Input: part model. Units: mm. Frame: model coordinates. Face numbers are marked on the shaded views. Coordinates: 2 decimals unless noted, no trailing zeros. Loops run counter-clockwise (first coordinate to the right, second up) from the corner with the lowest first, then second, coordinate; pieces in that order, holes last. Notation, with made-up numbers: (46.5, 26) -> (88.5, 26) arc R16 ccw to (88.5, 32) -> close; hole circle Ø3 at (29, 40). An arc over 180 degrees is marked (long way). Answer as a JSON object with one key per item and string values.
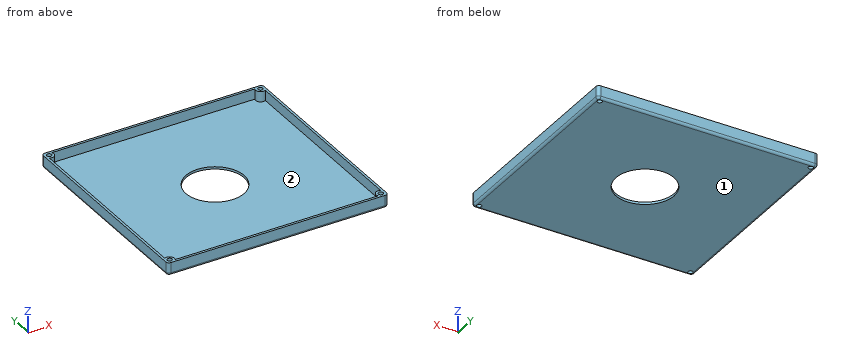
from build123d import *

# Parameters (mm, degrees)
SKETCH1_W                = 140
SKETCH1_H                = 133
BOSS_EXTRUDE1_DEPTH      = 8
F_3_0_3_DIAMETER_HOLE1_D = 3
SHELL3_T                 = -1.5
FILLET2_R                = 2
FILLET3_R                = 2
FILLET4_R                = 2
FILLET5_R                = 2
SKETCH13_R               = 18.454910332
CUT_EXTRUDE1_DEPTH       = 10
FILLET6_R                = 1.5


with BuildPart() as part:
    # Sketch1 → Boss-Extrude1 (new body)
    with BuildSketch(Plane.XY):
        Rectangle(SKETCH1_W, SKETCH1_H)
    extrude(amount=BOSS_EXTRUDE1_DEPTH)

    # Ø3.0 (3) Diameter Hole1 (through all)
    with Locations(Plane.XY.offset(8)):
        with Locations((-67, 63.5), (67, 63.5), (-67, -63.5), (67, -63.5)):
            Hole(F_3_0_3_DIAMETER_HOLE1_D / 2)

    # Shell3
    shell3_openings = [part.faces().sort_by_distance(p)[0] for p in [
        (0, 0, 8),
    ]]
    offset(amount=SHELL3_T, openings=shell3_openings)

    # Fillet2
    fillet2_edges = [part.edges().sort_by_distance(p)[0] for p in [
        (-70, 66.5, 4),
    ]]
    fillet(fillet2_edges, radius=FILLET2_R)

    # Fillet3
    fillet3_edges = [part.edges().sort_by_distance(p)[0] for p in [
        (-70, -66.5, 4),
    ]]
    fillet(fillet3_edges, radius=FILLET3_R)

    # Fillet4
    fillet4_edges = [part.edges().sort_by_distance(p)[0] for p in [
        (70, -66.5, 4),
    ]]
    fillet(fillet4_edges, radius=FILLET4_R)

    # Fillet5
    fillet5_edges = [part.edges().sort_by_distance(p)[0] for p in [
        (70, 66.5, 4),
    ]]
    fillet(fillet5_edges, radius=FILLET5_R)

    # Sketch13 → Cut-Extrude1 (cut)
    with BuildSketch(Plane(origin=(0, 0, 0), x_dir=(-1, 0, 0), z_dir=(0, 0, -1))):
        Circle(SKETCH13_R)
    extrude(amount=-CUT_EXTRUDE1_DEPTH, mode=Mode.SUBTRACT)

    # Fillet6
    fillet6_edges = [part.edges().sort_by_distance(p)[0] for p in [
        (-70, 0, 0),
        (-69.414213562, 65.914213562, 0),
        (0, -66.5, 0),
        (-69.414213562, -65.914213562, 0),
        (70, 0, 0),
        (69.414213562, -65.914213562, 0),
        (0, 66.5, 0),
        (69.414213562, 65.914213562, 0),
    ]]
    fillet(fillet6_edges, radius=FILLET6_R - 0.0001)  # a hair under: the kernel refuses the full size


solid = part.part
1. Section query A-A (y = -30). Return loops of the section in (x, z), plus the area to 3 significant figures.
Reply:
{"outline": "(-70, 1.5) arc R1.5 ccw to (-68.5, 0) -> (68.5, 0) arc R1.5 ccw to (70, 1.5) -> (70, 8) -> (68.5, 8) -> (68.5, 1.5) -> (-68.5, 1.5) -> (-68.5, 8) -> (-70, 8) -> close", "area": "229 mm2"}
2. Pin query (flat end, axial travel): P1, Ø22, axis at x = 0, y = 0, coming from the +Z side. Return the tip coordinate at first contact, or that it passes through.
Reply:
{"P1": "passes through"}
3. Section query D-D (x = 42.5). Return loops of the section in (y, z), plus the area to 3 significant figures.
Reply:
{"outline": "(-66.5, 1.5) arc R1.5 ccw to (-65, 0) -> (65, 0) arc R1.5 ccw to (66.5, 1.5) -> (66.5, 8) -> (65, 8) -> (65, 1.5) -> (-65, 1.5) -> (-65, 8) -> (-66.5, 8) -> close", "area": "218 mm2"}
4. Line query: line 1 along Y through (x, z) = (67, 2.75); line 2 along X through (y, z) = (-10.5, 4); line 3 along Y through (x, z) = (-19.5, 4.25). Output: solid intervals per line, ascending.
Reply:
{"line 1": "y = -66.5 to -65, -62 to -60.5, 60.5 to 62, 65 to 66.5", "line 2": "x = -70 to -68.5, 68.5 to 70", "line 3": "y = -66.5 to -65, 65 to 66.5"}
5. Section query B-B (z = 6.5). Return loops of the section in (x, y).
Reply:
{"outline": "(-70, -64.5) arc R2 ccw to (-68, -66.5) -> (68, -66.5) arc R2 ccw to (70, -64.5) -> (70, 64.5) arc R2 ccw to (68, 66.5) -> (-68, 66.5) arc R2 ccw to (-70, 64.5) -> close; hole circle Ø3 at (-67, -63.5); hole (-68.5, -60.9) arc R3 cw to (-64.4, -65) -> (64.4, -65) arc R3 cw to (68.5, -60.9) -> (68.5, 60.9) arc R3 cw to (64.4, 65) -> (-64.4, 65) arc R3 cw to (-68.5, 60.9) -> close; hole circle Ø3 at (-67, 63.5); hole circle Ø3 at (67, -63.5); hole circle Ø3 at (67, 63.5)"}
6. Section query C-C (x = 5). Return loops of the section in (y, z).
Reply:
{"outline": "(-66.5, 1.5) arc R1.5 ccw to (-65, 0) -> (-17.76, 0) -> (-17.76, 1.5) -> (-65, 1.5) -> (-65, 8) -> (-66.5, 8) -> close; (17.76, 0) -> (65, 0) arc R1.5 ccw to (66.5, 1.5) -> (66.5, 8) -> (65, 8) -> (65, 1.5) -> (17.76, 1.5) -> close"}
7. Mould query, pull axis X, two halves, no side actions, for the marked faces 1 and 2. Classes: pulls with the +X half, pulls with the -X half, needs draft (parallel to the pull), parting line crosses it, or undercut.
Reply:
{"face 1": "needs draft", "face 2": "undercut"}
